Part model, mm, in its own coordinate system. Give positions to 0.01 mm unless a question says otherwise; leave off trailing zeros. Order: outer loops, then holes, each group sorted by start corner. A loop starts at its lowest first (then second) coordinate and runs counter-clockwise, first axis right, second up.
1. Mould opens along X. For faces 1 (the flat face through (-25.4, 2, 3)), 2 (the flat face through (0, 3, 6.35)), 3 (the cylindrical face through (18.271, 182.982, 3.131)) say: +X half, -X half, draft (parallel to the pull), parting line (faces both ways), or undercut.
2. Probe line 1 (X direction, y = -110.5, z = 2.75); line 2 (Y direction, x = 5, z = 4.75); line 3 (Y direction, x = 0, z = 4.5). List the from-to ranges inside material, lowest first.
3. Slice it at A-A on z = 3. List the corners of the cut face in (x, y).
4. Slice it at B-B on x = 12.5. List the corners of the cut face in (y, z).
5. Drop a flat-ended pin along its axis: pin 1 Ø1 at (x, z) = (5, 4) entering from -Y. Give the stop position or say it passes through.
from build123d import *

# Parameters (mm, degrees)
F0_R     = 1.75
F0_R_2   = 2.55
F1_DEPTH = 6.35


with BuildPart() as f1:
    # F0 (on Top) → F1 (new body)
    with BuildSketch(Plane.XY):
        with BuildLine():
            ThreePointArc((25.4, 165.5), (18.07767, 183.17767), (0.4, 190.5))
            Line((0.4, 190.5), (-0.4, 190.5))
            ThreePointArc((-0.4, 190.5), (-18.07767, 183.17767), (-25.4, 165.5))
            Line((-25.4, 165.5), (-25.4, -165.5))
            ThreePointArc((-25.4, -165.5), (-18.07767, -183.17767), (-0.4, -190.5))
            Line((-0.4, -190.5), (0.4, -190.5))
            ThreePointArc((0.4, -190.5), (18.07767, -183.17767), (25.4, -165.5))
            Line((25.4, -165.5), (25.4, 165.5))
        make_face()
        with Locations((-5, -160.5)):
            Circle(F0_R, mode=Mode.SUBTRACT)
        with Locations((-5, -110.5)):
            Circle(F0_R, mode=Mode.SUBTRACT)
        with Locations((5, -160.5)):
            Circle(F0_R, mode=Mode.SUBTRACT)
        with Locations((5, -110.5)):
            Circle(F0_R, mode=Mode.SUBTRACT)
        with Locations((0, 170.5)):
            Circle(F0_R_2, mode=Mode.SUBTRACT)
    extrude(amount=F1_DEPTH)


solid = f1.part
Data:
1. face 1: -X half
1. face 2: draft
1. face 3: +X half
2. line 1: x = -25.4 to -6.75, -3.25 to 3.25, 6.75 to 25.4
2. line 2: y = -190.07 to -162.25, -158.75 to -112.25, -108.75 to 190.07
2. line 3: y = -190.5 to 167.95, 173.05 to 190.5
3. outline: (-25.4, -165.5) arc R25 ccw to (-0.4, -190.5) - (0.4, -190.5) arc R25 ccw to (25.4, -165.5) - (25.4, 165.5) arc R25 ccw to (0.4, 190.5) - (-0.4, 190.5) arc R25 ccw to (-25.4, 165.5) - close; hole circle Ø3.5 at (-5, -160.5); hole circle Ø3.5 at (-5, -110.5); hole circle Ø5.1 at (0, 170.5); hole circle Ø3.5 at (5, -160.5); hole circle Ø3.5 at (5, -110.5)
4. outline: (-187.38, 0) - (187.38, 0) - (187.38, 6.35) - (-187.38, 6.35) - close
5. pin 1: stops at y = -190.16
